from build123d import *

# Parameters (mm, degrees)
SKETCH_1_R          = 6.45
EXTRUDE_1_DEPTH     = 1
SKETCH_2_W          = 1.693962672
SKETCH_2_H          = 6.211196465
CUT_EXTRUDE_1_DEPTH = 10


with BuildPart() as part:
    # 草图1 → 凸台-拉伸1 (new body)
    with BuildSketch(Plane(origin=(0, 0, 0), x_dir=(1, 0, 0), z_dir=(0, 1, 0))):
        with BuildLine():
            Line((0, -9.465309979), (2, -9.465309979))
            Line((2, -9.465309979), (3, -6.754136751))
            ThreePointArc((3, -6.754136751), (0, 8.35), (-3, -6.754136751))
            Line((-3, -6.754136751), (-2, -9.465309979))
            Line((-2, -9.465309979), (0, -9.465309979))
        make_face()
        with Locations(Location((0, 0, 0), (0, 0, 270))):
            Circle(SKETCH_1_R, mode=Mode.SUBTRACT)
    extrude(amount=EXTRUDE_1_DEPTH)

    # 草图2 → 切除-拉伸1 (cut)
    with BuildSketch(Plane(origin=(0, 1, 0), x_dir=(1, 0, 0), z_dir=(0, 1, 0))):
        with Locations((-0.053964614, -8.617371485)):
            Rectangle(SKETCH_2_W, SKETCH_2_H)
    extrude(amount=-CUT_EXTRUDE_1_DEPTH, mode=Mode.SUBTRACT)


solid = part.part
CAD build for the part. Positions are in the model's coordinates, mm. A direction names the side the tool comes from. Round coordinates to 2 decimals unless told otherwise and drop trailing zeros. Order: outer loops, then holes, each group sorted by start corner. A loop starts at its lowest first (then second) coordinate and runs counter-clockwise, first axis right, second up. Notation, with made-up numbers: M 76,14 L 95,14 A20 cw 95,37 Z; hole C 52,53.5 d9. An arc over 180 degrees is marked long. Use one line per item in the form item = value.
Q1. Flat gauge pin, fed straight in: P1, Ø7.5, axis at x = 0, z = 0, coming from the +Y side. Where does the tip first touch, or does it go through?
Recorded:
P1 = through
Q2. Saw through at C-C on y = 0.7. Give the cut face in (x, z).
Recorded:
outline = M -3,6.75 A7.85 ccw long 3,6.75 L 2,9.47 L 0.79,9.47 L 0.79,6.4 A6.45 cw long -0.9,6.39 L -0.9,9.47 L -2,9.47 Z
Q3. Probe L1, parallel to X at y = 0.2, z = 0; L2, parallel to X at y = 0.65, z = 2.5; L3, parallel to Z at x = -1.25, y = 0.15. List the from-to ranges inside material, lowest first.
Recorded:
L1 = -7.83 to -6.45, 6.45 to 7.83
L2 = -7.25 to -5.95, 5.95 to 7.25
L3 = -8.25 to -6.33, 6.33 to 9.47
Q4. Two-plate mould, pull along X, no slides. Class faces 3 (the flat face through (1.4, 0.5, 9.465)), 4 (the cylindrical face through (0.302, 0.493, -8.344)), 5 (the flat face through (-0.901, 0.5, 7.9)): +X half, -X half, draft (parallel to the pull), parting line (faces both ways), or undercut.
Recorded:
face_3 = draft
face_4 = parting line
face_5 = undercut
Q5. Saw through at A-A on x = -2.25. Give the cut face in (y, z), then the cut area to 3 significant figures.
Recorded:
outline = M 0,-8.02 L 1,-8.02 L 1,-6.04 L 0,-6.04 Z; M 0,6.04 L 1,6.04 L 1,8.79 L 0,8.79 Z
area = 4.72 mm^2
Q6. Saw through at B-B on z = -6. Give the cut face in (x, y), then the cut area to 3 significant figures.
Recorded:
outline = M -5.6,0 L -2.37,0 L -2.37,1 L -5.6,1 Z; M 2.37,0 L 5.6,0 L 5.6,1 L 2.37,1 Z
area = 6.47 mm^2
Q7. Which spindle directions (+Z, -Z, +X, -X, +Y, -Y) get a long thin tool onto all of the face, cutting with end or side? Do faces 1 (the flat face through (2.493, 0.493, 8.129)), 2 (the flat face through (0.793, 0.5, 8)). Say none if no direction does.
Recorded:
face_1 = +Z, +X, +Y, -Y
face_2 = +Z, +Y, -Y
Q8. Saw through at D-D on x = 0. Give the cut face in (y, z), then the cut area to 3 significant figures.
Recorded:
outline = M 0,-8.35 L 1,-8.35 L 1,-6.45 L 0,-6.45 Z
area = 1.90 mm^2
